For this review, take the finished solid that the model builds, in its own axes (mm). A direction names the side the tool comes from. Give positions to 0.01 mm unless a question says otherwise; leave off trailing zeros. Write each loop counter-clockwise with the first axis right and the second up, starting at its lowest first coordinate (ties: lowest second). Pieces come first, ordered by that corner, then holes. Notation, with made-up numbers: M 57.25,-38.75 L 65.25,-38.75 A18 ccw 65.25,-6.75 Z; hole C -3,-25.5 d10. An arc over 180 degrees is marked long. One line per item, written item: value. Start each with the question number.
Item 1: Mouldability with a two-part tool opening along X and no side actions: class faces 1 (the face through (18.844, 0.123, 9.392)), 2 (the face through (26.558, 0, -32)), 3 (the face through (-26.782, 0, -32)) as released by +X, released by -X, zero draft, split by the parting line, or undercut.
Item 2: To check wall thickness, follow probe 1 along Z at (x, y) = (13, -4.75); probe 2 along Z at (x, y) = (1, -0.5); probe 3 along Z at (x, y) = (8.5, -0.5). State the ranges of each line that lie inside material, in increasing order.
Item 3: Consider section D-D, the plane x = 23.5. Write out the cut boundary in (y, z), and give its area (3 significant figures).
Item 4: Consider section C-C, the plane z = -31. Write out the cut boundary in (x, y), and give its area (3 significant figures).
Item 5: Tool access review of faces 4 (the face through (-18.844, 0.123, 9.658)), 5 (the face through (-25.333, -7.362, -31.306)): name each direction out of +Z, -Z, +X, -X, +Y, -Y from which nothing blocks a thin tool from reaching the whole face with its end or side.
Item 6: Clearance check with flat-ended pins moving along their axes: pin 1 Ø8 at (x, y) = (-12, -3.5) entering from +Z; pin 2 Ø9 at (x, y) = (-1.5, -0.5) entering from +Z; pin 3 Ø6 at (y, z) = (0, 3.5) entering from -X. State where each tip first meets the part, or that it passes through.
Item 7: Consider section B-B, the plane z = 12. Write out the cut boundary in (x, y), and give its area (3 significant figures).
Item 8: Consider section A-A, the plane y = 0. Write out the cut boundary in (x, z).
```python
from build123d import *

# Parameters (mm, degrees)
F1_R     = 2.794
F3_W     = 53.34
F3_H     = 63.5
F4_DEPTH = 8.89
F5_R     = 5.08


with BuildPart() as f2:
    # F2: sweep along a path in F0
    with BuildLine(Plane.XZ) as f2_path:
        Line((-16.0525806478, 0), (-16.0525806478, 19.05))
        ThreePointArc((-16.0525806478, 19.05), (0, 35.1025806478), (16.0525806478, 19.05))
        Line((16.0525806478, 19.05), (16.0525806478, 0))
    # F1 (on Top) → F2 (sweep)
    with BuildSketch(Plane.XY):
        with Locations((-16.0525806478, 0)):
            Circle(F1_R)
    sweep(path=f2_path.line)

    # F3 (on Front) → F4 (join, symmetric)
    with BuildSketch(Plane.XZ):
        with Locations((-0.1116646679, -31.75)):
            Rectangle(F3_W, F3_H)
    extrude(amount=F4_DEPTH, both=True)

    # F5
    f5_edges = [f2.edges().sort_by_distance(p)[0] for p in [
        (-26.781665, -8.89, -31.75),
        (-26.781665, 8.89, -31.75),
        (26.558335, 8.89, -31.75),
        (26.558335, -8.89, -31.75),
    ]]
    fillet(f5_edges, radius=F5_R)


solid = f2.part
```
Model answer:
1. face 1: undercut
1. face 2: released by +X
1. face 3: released by -X
2. probe 1: z = -63.5 to 0
2. probe 2: z = -63.5 to 0, 32.32 to 37.82
2. probe 3: z = -63.5 to 0, 29.28 to 35.82
3. outline: M -8.47,-63.5 L 8.47,-63.5 L 8.47,0 L -8.47,0 Z
3. area: 1,080 mm2
4. outline: M -26.78,-3.81 A5.08 ccw -21.7,-8.89 L 21.48,-8.89 A5.08 ccw 26.56,-3.81 L 26.56,3.81 A5.08 ccw 21.48,8.89 L -21.7,8.89 A5.08 ccw -26.78,3.81 Z
4. area: 926 mm2
5. face 4: none
5. face 5: +Z, -Z, -X, -Y
6. pin 1: stops at z = 35.46
6. pin 2: stops at z = 37.9
6. pin 3: stops at x = -18.85
7. outline: C -16.05,0 d5.59; C 16.05,0 d5.59
7. area: 49.0 mm2
8. outline: M -26.78,-63.5 L 26.56,-63.5 L 26.56,0 L 18.85,0 L 18.85,19.05 A18.85 ccw -18.85,19.05 L -18.85,0 L -26.78,0 Z; hole M -13.26,0 L 13.26,0 L 13.26,19.05 A13.26 ccw -13.26,19.05 Z
